Design review of the part built by this model. Coordinates are the model's own, in mm. A direction names the side the tool comes from. Give positions to 0.01 mm unless a question says otherwise; leave off trailing zeros. Loops run counter-clockwise (first coordinate to the right, second up) from the corner with the lowest first, then second, coordinate; pieces in that order, holes last. Notation, with made-up numbers: M 80.5,-8 L 94.5,-8 A9 ccw 94.5,3 Z; hole C -19.5,63.25 d5. An arc over 180 degrees is marked long. Use a Markdown table: item, result. Add a question column.
(1) Add section A-A, the plane z = -26.08. Give the boundary of the cut face in (x, y) (3 decimals), then the cut area to 3 significant figures.
(2) Insertion check: pin 1 Ø4 at (y, z) = (0, -40) entering from +X; pin 2 Ø6 at (x, z) = (2.5, -8.5) entering from +Y (3 decimals); pin 3 Ø0.5 at (y, z) = (9, -17.5) entering from -X; pin 4 Ø6 at (y, z) = (-4, -13.5) entering from +X. Each pin has a flat end and moves straight along its axis. Give the tip position at first contact, or say it passes through.
(3) Add section C-C, the plane y = 0. State how many separate pieces and enclosed holes the cut face has, then the cut area to 3 significant figures.
(4) Add section D-D, the plane z = -39.4. Give the boundary of the cut face in (x, y).
(5) Add section B-B, the plane z = -19. Give the boundary of the cut face in (x, y) (3 decimals).
(6) Draft analysis for pull direction Z (two halves, no side actions). For faces 1 (the face through (-7.92, -9.1, -17.5)), 2 (the face through (0, -10.053, -18)), 3 (the face through (-9.681, 0.056, 8.096)), 4 (the face through (-10.1, 3.5, 7.1)), state which applies: pulls with the +Z half, pulls with the -Z half, needs draft (parallel to the pull), parting line crosses it, or undercut.
(7) For faces 5 (the face through (-1.4, 0, -37.8)), 6 (the face through (-5.062, 9.052, 5.185)), 7 (the face through (10.1, 3.5, 7.1)), 8 (the face through (-9, 0, 7.35)), list the 3-axis set-ups (+Z, -Z, +X, -X, +Y, -Y) from which the entire face can be reached by the end or side of a thin tool; tool diameter is ignored.
(8) For probe 1 along X at (y, z) = (5, -0.5); probe 2 along Y at (x, z) = (-0.25, -18.5) (3 decimals); probe 3 along Z at (x, y) = (-6.25, 3.25), list the stretches that pass through material, from the lowest coordinate up.
```python
from build123d import *

# Parameters (mm, degrees)
BOSS_EXTRUDE1_DEPTH  = 11.2
BOSS_EXTRUDE2_DEPTH  = 1
BOSS_EXTRUDE4_DEPTH  = 36
SKETCH5_W            = 8.920001513
SKETCH5_H            = 22.167921158
BOSS_EXTRUDE6_DEPTH  = 2
FILLET2_R            = 5
SKETCH6_W            = 1.4
SKETCH6_H            = 5
BOSS_EXTRUDE7_DEPTH  = 4.8
SKETCH7_R            = 1.38
CUT_EXTRUDE1_DEPTH   = 4.8
SKETCH8_R            = 3.675
SKETCH8_R_2          = 3.175
BOSS_EXTRUDE8_DEPTH  = 0.5
SKETCH9_R            = 3.175
CUT_EXTRUDE2_DEPTH   = 7.5
CHAMFER1_SIZE        = 1
SKETCH10_R           = 1.845
BOSS_EXTRUDE9_DEPTH  = 1.92
CHAMFER2_SIZE        = 0.5
SKETCH11_R           = 1.5
CUT_EXTRUDE3_DEPTH   = 1.92
SKETCH12_R           = 1.15
CUT_EXTRUDE4_DEPTH   = 1.92
BOSS_EXTRUDE13_DEPTH = 0.5
SKETCH14_W           = 3.5
SKETCH14_H           = 7
CUT_EXTRUDE6_DEPTH   = 5.5
BOSS_EXTRUDE14_DEPTH = 7
SKETCH16_W           = 0.5
SKETCH16_H           = 7
BOSS_EXTRUDE16_DEPTH = 2
CHAMFER3_SIZE        = 0.5
SKETCH20_R           = 0.5
BOSS_EXTRUDE19_DEPTH = 15
SKETCH21_R           = 1.5
SKETCH21_R_2         = 1.237971005
SKETCH21_R_3         = 1.15
SKETCH21_R_4         = 0.940138742
BOSS_EXTRUDE23_DEPTH = 1
SKETCH21_2_R         = 1.5
SKETCH21_2_R_2       = 1.237971005
SKETCH21_2_R_3       = 1.15
SKETCH21_2_R_4       = 0.940138742
BOSS_EXTRUDE24_DEPTH = 8
SKETCH22_R           = 0.8
SKETCH22_R_2         = 0.5
BOSS_EXTRUDE25_DEPTH = 8
FILLET4_R            = 0.5


with BuildPart() as part:
    # Sketch1 → Boss-Extrude1 (new body)
    with BuildSketch(Plane.XY):
        with BuildLine():
            Line((0, 11.115), (0, 10.171175948))
            Line((0, 10.171175948), (-1, 10.171175948))
            ThreePointArc((-1, 10.171175948), (-5.011187662, 9.081675078), (-7.920001513, 6.112594314))
            Line((-7.920001513, 6.112594314), (-7.920001513, -6.112594314))
            ThreePointArc((-7.920001513, -6.112594314), (-5.011187662, -9.081675078), (-1, -10.171175948))
            Line((-1, -10.171175948), (0, -10.171175948))
            Line((0, -10.171175948), (0, -11.115))
            ThreePointArc((0, -11.115), (-5.196692773, -10.123430296), (-8.920001513, -6.365))
            Line((-8.920001513, -6.365), (-8.920001513, 6.365))
            ThreePointArc((-8.920001513, 6.365), (-5.196692773, 10.123430296), (0, 11.115))
        make_face()
    extrude(amount=BOSS_EXTRUDE1_DEPTH)

    # Sketch2 → Boss-Extrude2 (add)
    with BuildSketch(Plane(origin=(0, 0, 0), x_dir=(-1, 0, 0), z_dir=(0, 0, -1))):
        with BuildLine():
            Line((2, 11.115), (8.920001513, 11.115))
            Line((8.920001513, 11.115), (8.920001513, -11.052921158))
            Line((8.920001513, -11.052921158), (2.44835684, -11.052921158))
            ThreePointArc((2.44835684, -11.052921158), (1.226317056, -11.16830724), (0, -11.115))
            Line((0, -11.115), (0, -10.171175948))
            Line((0, -10.171175948), (1, -10.171175948))
            ThreePointArc((1, -10.171175948), (5.011187662, -9.081675078), (7.920001513, -6.112594314))
            Line((7.920001513, -6.112594314), (7.920001513, 6.112594314))
            ThreePointArc((7.920001513, 6.112594314), (5.011187662, 9.081675078), (1, 10.171175948))
            Line((1, 10.171175948), (0, 10.171175948))
            Line((0, 10.171175948), (0, 11.115))
            ThreePointArc((0, 11.115), (1, 11.171175948), (2, 11.115))
        make_face()
    extrude(amount=BOSS_EXTRUDE2_DEPTH)

    # Sketch4 → Boss-Extrude4 (add)
    with BuildSketch(Plane(origin=(0, 0, -1), x_dir=(-1, 0, 0), z_dir=(0, 0, -1))):
        Polygon((8.920001513, 11.115), (0, 11.115), (0, 10.115), (1, 10.115), (7.920001513, 10.115), (7.920001513, -10.052921158), (1, -10.052921158), (0, -10.052921158), (0, -11.052921158), (8.920001513, -11.052921158), align=None)
    extrude(amount=BOSS_EXTRUDE4_DEPTH)

    # Sketch5 → Boss-Extrude6 (add)
    with BuildSketch(Plane(origin=(0, 0, -37), x_dir=(-1, 0, 0), z_dir=(0, 0, -1))):
        with Locations((4.460000757, 0.031039421)):
            Rectangle(SKETCH5_W, SKETCH5_H)
    extrude(amount=-BOSS_EXTRUDE6_DEPTH)

    # Fillet2
    fillet2_edges = [part.edges().sort_by_distance(p)[0] for p in [
        (-3.960000757, 10.115, -35),
        (-4.460000757, 11.115, -37),
        (-4.460000757, -11.052921158, -37),
        (-3.960000757, -10.052921158, -35),
    ]]
    fillet(fillet2_edges, radius=FILLET2_R)

    # Sketch6 → Boss-Extrude7 (add)
    with BuildSketch(Plane(origin=(0, 0, -37), x_dir=(-1, 0, 0), z_dir=(0, 0, -1))):
        with Locations((0.7, 0)):
            Rectangle(SKETCH6_W, SKETCH6_H)
    extrude(amount=BOSS_EXTRUDE7_DEPTH)

    # Sketch7 → Cut-Extrude1 (cut)
    with BuildSketch(Plane.ZY.offset(1.4)):
        with Locations((-39.4, 0)):
            Circle(SKETCH7_R)
    extrude(amount=-CUT_EXTRUDE1_DEPTH, mode=Mode.SUBTRACT)

    # Sketch8 → Boss-Extrude8 (add)
    with BuildSketch(Plane.ZY.offset(8.920001513)):
        with Locations((-26.08, 0)):
            Circle(SKETCH8_R)
        with Locations((-26.08, 0)):
            Circle(SKETCH8_R_2, mode=Mode.SUBTRACT)
    extrude(amount=BOSS_EXTRUDE8_DEPTH)

    # Sketch9 → Cut-Extrude2 (cut)
    with BuildSketch(Plane.ZY.offset(8.920001513)):
        with Locations((-26.08, 0)):
            Circle(SKETCH9_R)
    extrude(amount=-CUT_EXTRUDE2_DEPTH, mode=Mode.SUBTRACT)

    # Chamfer1
    chamfer1_edges = [part.edges().sort_by_distance(p)[0] for p in [
        (-0.7, -2.5, -37),
        (-0.7, 2.5, -37),
    ]]
    chamfer(chamfer1_edges, length=CHAMFER1_SIZE)

    # Sketch10 → Boss-Extrude9 (add)
    with BuildSketch(Plane.ZY.offset(8.920001513)):
        with Locations((-14.83, 0)):
            Circle(SKETCH10_R)
    extrude(amount=BOSS_EXTRUDE9_DEPTH)

    # Chamfer2
    chamfer2_edges = [part.edges().sort_by_distance(p)[0] for p in [
        (-10.840001513, 0, -16.675),
    ]]
    chamfer(chamfer2_edges, length=CHAMFER2_SIZE)

    # Sketch11 → Cut-Extrude3 (cut)
    with BuildSketch(Plane.ZY.offset(8.920001513)):
        with Locations((-5.83, 8.71)):
            Circle(SKETCH11_R)
        with Locations((-5.83, -8.71)):
            Circle(SKETCH11_R)
    extrude(amount=-CUT_EXTRUDE3_DEPTH, mode=Mode.SUBTRACT)

    # Sketch12 → Cut-Extrude4 (cut)
    with BuildSketch(Plane.ZY.offset(8.920001513)):
        with Locations((-3.140037022, 7.781512681)):
            Circle(SKETCH12_R)
        with Locations((-3.140037022, -7.781512681)):
            Circle(SKETCH12_R)
    extrude(amount=-CUT_EXTRUDE4_DEPTH, mode=Mode.SUBTRACT)

    # Sketch13 → Boss-Extrude13 (add)
    with BuildSketch(Plane(origin=(0, 0, -1), x_dir=(-1, 0, 0), z_dir=(0, 0, -1))):
        with BuildLine():
            Line((7.920001513, 10.115), (0, 10.115))
            Line((0, 10.115), (0, 2.5))
            ThreePointArc((0, 2.5), (2.5, 0), (0, -2.5))
            Line((0, -2.5), (0, -10.115))
            Line((0, -10.115), (0, -10.171175948))
            Line((0, -10.171175948), (0.5, -10.171175948))
            Line((0.5, -10.171175948), (7.920001513, -10.171175948))
            Line((7.920001513, -10.171175948), (7.920001513, 10.115))
        make_face()
    extrude(amount=BOSS_EXTRUDE13_DEPTH)

    # Sketch14 → Cut-Extrude6 (cut)
    with BuildSketch(Plane.ZY.offset(8.920001513)):
        with Locations((5.6, 0)):
            Rectangle(SKETCH14_W, SKETCH14_H)
    extrude(amount=-CUT_EXTRUDE6_DEPTH, mode=Mode.SUBTRACT)

    # Sketch15 → Boss-Extrude14 (add)
    with BuildSketch(Plane.XZ.offset(-3.5)):
        Polygon((-8.920001513, 7.35), (-10.420001513, 7.35), (-10.420001513, 7.85), (-8.920001513, 8.35), align=None)
    extrude(amount=BOSS_EXTRUDE14_DEPTH)

    # Sketch16 → Boss-Extrude16 (add)
    with BuildSketch(Plane(origin=(0, 0, 7.35), x_dir=(-1, 0, 0), z_dir=(0, 0, -1))):
        with Locations((10.170001513, 0)):
            Rectangle(SKETCH16_W, SKETCH16_H)
    extrude(amount=BOSS_EXTRUDE16_DEPTH)

    # Chamfer3
    chamfer3_edges = [part.edges().sort_by_distance(p)[0] for p in [
        (-8.920001513, 3.5, 7.85),
        (-8.920001513, -3.5, 7.85),
    ]]
    chamfer(chamfer3_edges, length=CHAMFER3_SIZE)

    # Sketch20 → Boss-Extrude19 (add)
    with BuildSketch(Plane(origin=(-7.920001513, 0, 0), x_dir=(0, 0, -1), z_dir=(1, 0, 0))):
        with Locations((16.425, 0)):
            Circle(SKETCH20_R)
    extrude(amount=BOSS_EXTRUDE19_DEPTH)

    # Sketch21 → Boss-Extrude23 (add)
    with BuildSketch(Plane(origin=(-7.920001513, 0, 0), x_dir=(0, 0, -1), z_dir=(1, 0, 0))):
        with Locations((5.83, 8.71)):
            Circle(SKETCH21_R)
        with Locations((5.83, 8.71)):
            Circle(SKETCH21_R_2, mode=Mode.SUBTRACT)
        with Locations((3.140037022, 7.781512681)):
            Circle(SKETCH21_R_3)
        with Locations((3.140037022, 7.781512681)):
            Circle(SKETCH21_R_4, mode=Mode.SUBTRACT)
        with Locations((3.140037022, -7.781512681)):
            Circle(SKETCH21_R_3)
        with Locations((3.140037022, -7.781512681)):
            Circle(SKETCH21_R_4, mode=Mode.SUBTRACT)
        with Locations((5.83, -8.71)):
            Circle(SKETCH21_R)
        with Locations((5.83, -8.71)):
            Circle(SKETCH21_R_2, mode=Mode.SUBTRACT)
    extrude(amount=-BOSS_EXTRUDE23_DEPTH)

    # Sketch21_2 → Boss-Extrude24 (add)
    with BuildSketch(Plane(origin=(-7.920001513, 0, 0), x_dir=(0, 0, -1), z_dir=(1, 0, 0))):
        with Locations((5.83, 8.71)):
            Circle(SKETCH21_2_R)
        with Locations((5.83, 8.71)):
            Circle(SKETCH21_2_R_2, mode=Mode.SUBTRACT)
        with Locations((3.140037022, 7.781512681)):
            Circle(SKETCH21_2_R_3)
        with Locations((3.140037022, 7.781512681)):
            Circle(SKETCH21_2_R_4, mode=Mode.SUBTRACT)
        with Locations((3.140037022, -7.781512681)):
            Circle(SKETCH21_2_R_3)
        with Locations((3.140037022, -7.781512681)):
            Circle(SKETCH21_2_R_4, mode=Mode.SUBTRACT)
        with Locations((5.83, -8.71)):
            Circle(SKETCH21_2_R)
        with Locations((5.83, -8.71)):
            Circle(SKETCH21_2_R_2, mode=Mode.SUBTRACT)
    extrude(amount=BOSS_EXTRUDE24_DEPTH)

    # Sketch22 → Boss-Extrude25 (add)
    with BuildSketch(Plane(origin=(-7.920001513, 0, 0), x_dir=(0, 0, -1), z_dir=(1, 0, 0))):
        with Locations((17.526449978, 9.081390514)):
            Circle(SKETCH22_R)
        with Locations((17.526449978, 9.081390514)):
            Circle(SKETCH22_R_2, mode=Mode.SUBTRACT)
        with Locations((31.797803684, 8.592263442)):
            Circle(SKETCH22_R)
        with Locations((31.797803684, 8.592263442)):
            Circle(SKETCH22_R_2, mode=Mode.SUBTRACT)
        with Locations((31.797803684, -8.592263442)):
            Circle(SKETCH22_R)
        with Locations((31.797803684, -8.592263442)):
            Circle(SKETCH22_R_2, mode=Mode.SUBTRACT)
        with Locations((17.526449978, -9.081390514)):
            Circle(SKETCH22_R)
        with Locations((17.526449978, -9.081390514)):
            Circle(SKETCH22_R_2, mode=Mode.SUBTRACT)
    extrude(amount=BOSS_EXTRUDE25_DEPTH)

    # Mirror7: part across plane


with BuildPart() as part_1:
    add(part.part)
    add(part.part.mirror(Plane(origin=(0, 0, 0), x_dir=(0, 0, 1), z_dir=(1, 0, 0))))

    # Fillet4
    fillet4_edges = [part_1.edges().sort_by_distance(p)[0] for p in [
        (-8.920001513, 0.031039421, -37),
        (-8.920001513, -11.052921158, -16),
        (-8.920001513, 11.115, -16),
        (-8.920001513, 9.650533906, -35.535533906),
        (-8.920001513, -9.588455064, -35.535533906),
        (8.920001513, 0.031039421, -37),
        (8.920001513, 11.115, -16),
        (8.920001513, -11.052921158, -16),
        (8.920001513, -9.588455064, -35.535533906),
        (8.920001513, 9.650533906, -35.535533906),
    ]]
    fillet(fillet4_edges, radius=FILLET4_R)


solid = part_1.part
```
Established:
| question | item | result |
|---|---|---|
| 1 | outline | M -9.42,-3.675 L -8.92,-3.675 L -8.92,-10.553 A0.5 ccw -8.42,-11.053 L 8.42,-11.053 A0.5 ccw 8.92,-10.553 L 8.92,-3.675 L 9.42,-3.675 L 9.42,-3.175 L 7.92,-3.175 L 7.92,-10.053 L -7.92,-10.053 L -7.92,-3.175 L -9.42,-3.175 Z; M -9.42,3.175 L -7.92,3.175 L -7.92,10.115 L 7.92,10.115 L 7.92,3.175 L 9.42,3.175 L 9.42,3.675 L 8.92,3.675 L 8.92,10.615 A0.5 ccw 8.42,11.115 L -8.42,11.115 A0.5 ccw -8.92,10.615 L -8.92,3.675 L -9.42,3.675 Z |
| 1 | area | 64.1 mm^2 |
| 2 | pin 1 | x = 1.4 |
| 2 | pin 2 | y = 11.115 |
| 2 | pin 3 | x = -8.92 |
| 2 | pin 4 | x = 10.84 |
| 3 | separate pieces | 5 |
| 3 | enclosed holes | 0 |
| 3 | area | 154 mm^2 |
| 4 | outline | M -1.4,-2.5 L 1.4,-2.5 L 1.4,-1.38 L -1.4,-1.38 Z; M -1.4,1.38 L 1.4,1.38 L 1.4,2.5 L -1.4,2.5 Z |
| 5 | outline | M -8.92,-10.553 A0.5 ccw -8.42,-11.053 L 8.42,-11.053 A0.5 ccw 8.92,-10.553 L 8.92,10.615 A0.5 ccw 8.42,11.115 L -8.42,11.115 A0.5 ccw -8.92,10.615 Z; hole M -7.92,-10.053 L 7.92,-10.053 L 7.92,10.115 L -7.92,10.115 Z |
| 6 | face 1 | undercut |
| 6 | face 2 | undercut |
| 6 | face 3 | pulls with the +Z half |
| 6 | face 4 | needs draft |
| 7 | face 5 | -Z, -X, +Y, -Y |
| 7 | face 6 | +Z |
| 7 | face 7 | +Z, -Z, +X, +Y |
| 7 | face 8 | none |
| 8 | probe 1 | -8.92 to -7.92, 7.92 to 8.92 |
| 8 | probe 2 | -11.053 to -10.053, 10.115 to 11.115 |
| 8 | probe 3 | -37 to -35, -1.5 to -1 |
